Answer from the drawing. Dimensions are ordinates in mm from the lowest x, y and z of the part. Round coordinates to 2 decimals unless told otherwise and drop trailing zeros. Order: outer loops, then holes, each group sorted by start corner. A loop starts at its lowest first (then second) coordinate and runs counter-clockwise, first axis right, second up.
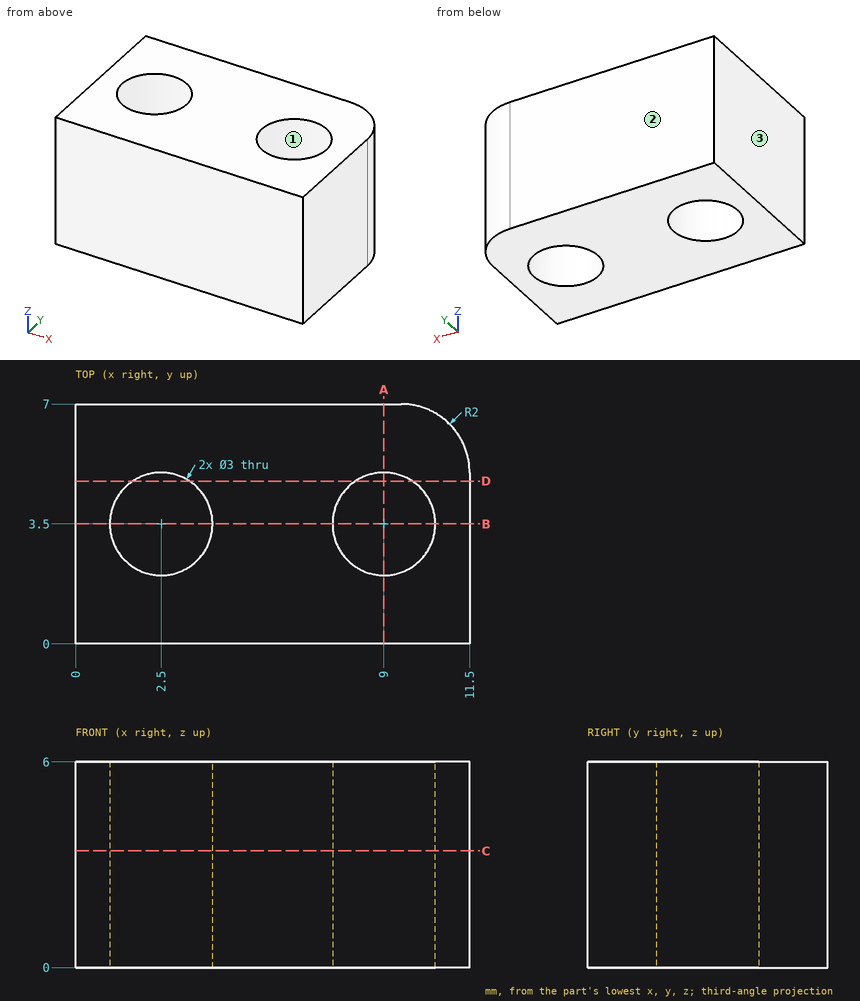
Q1. A cutting plane is placed at B-B, the plane y = 3.5. Give the vertices of the cut face in (x, z), plus the area to 3 significant figures.
Outcome:
outline: (0, 0) - (1, 0) - (1, 6) - (0, 6) - close; (4, 0) - (7.5, 0) - (7.5, 6) - (4, 6) - close; (10.5, 0) - (11.5, 0) - (11.5, 6) - (10.5, 6) - close
area: 33.0 mm2
Q2. Straight lines are drawn through the part: probe 1 along Y at (x, z) = (9, 2.75); probe 2 along Y at (x, z) = (8.25, 1.5). For each, find the intervals that lie inside material, in ascending order.
Outcome:
probe 1: y = 0 to 2, 5 to 7
probe 2: y = 0 to 2.2, 4.8 to 7
Q3. A cutting plane is placed at C-C, the plane z = 3.4. Give the vertices of the cut face in (x, y).
Outcome:
outline: (0, 0) - (11.5, 0) - (11.5, 5) arc R2 ccw to (9.5, 7) - (0, 7) - close; hole circle Ø3 at (2.5, 3.5); hole circle Ø3 at (9, 3.5)
Q4. Flat-ended cylindrical pins translate along their axes: pin 1 (1.8 mm diameter, centred on x = 9, y = 3.5, fed in from -Z); pin 2 (1 mm diameter, centred on y = 5.5, z = 5.5, fed in from -X). Find the tip coordinate at first contact, or state that the pin passes through.
Outcome:
pin 1: passes through
pin 2: stops at x = 0
Q5. For a pull along Y with two mould halves and no side action, classify the marked faces 1, 2 and 3 as released by +Y, released by -Y, zero draft, split by the parting line, or undercut.
Outcome:
face 1: undercut
face 2: released by +Y
face 3: zero draft
Q6. A cutting plane is placed at A-A, the plane x = 9. Give the vertices of the cut face in (y, z), plus the area to 3 significant figures.
Outcome:
outline: (0, 0) - (2, 0) - (2, 6) - (0, 6) - close; (5, 0) - (7, 0) - (7, 6) - (5, 6) - close
area: 24.0 mm2
Q7. A cutting plane is placed at D-D, the plane y = 4.75. Give the vertices of the cut face in (x, z), plus the area to 3 significant figures.
Outcome:
outline: (0, 0) - (1.67, 0) - (1.67, 6) - (0, 6) - close; (3.33, 0) - (8.17, 0) - (8.17, 6) - (3.33, 6) - close; (9.83, 0) - (11.5, 0) - (11.5, 6) - (9.83, 6) - close
area: 49.1 mm2
